```python
from build123d import *

# Parameters (mm, degrees)
F0_R     = 18.25
F0_R_2   = 16.25
F1_DEPTH = 2
F3_DEPTH = 1
F4_R     = 0.99999


# Not quite as in the source:
# - a fillet or chamfer is up to 0.001 mm smaller than in the source, because OpenCascade refuses the exact size


with BuildPart() as f1:
    # F0 (on Top) → F1 (new body)
    with BuildSketch(Plane.XY):
        Circle(F0_R)
        Circle(F0_R_2, mode=Mode.SUBTRACT)
    extrude(amount=F1_DEPTH)

    # F2 (on face) → F3 (join)
    with BuildSketch(Plane.XY.offset(2)):
        with BuildLine():
            ThreePointArc((-13.6956579083, 8.7459393126), (-12.9247475177, 8.70670819), (-12.5275195769, 9.368563064))
            ThreePointArc((-12.5275195769, 9.368563064), (-12.6077000662, 9.7059676033), (-12.8310977719, 9.9712301131))
            ThreePointArc((-12.8310977719, 9.9712301131), (-13.2775195769, 9.368563064), (-13.6956579083, 8.7459393126))
        make_face()
        with BuildLine():
            ThreePointArc((-13.6956579083, 8.7459393126), (-13.2775195769, 9.368563064), (-12.8310977719, 9.9712301131))
            ThreePointArc((-12.8310977719, 9.9712301131), (-13.8903281728, 9.8009582824), (-13.6956579083, 8.7459393126))
        make_face()
        with BuildLine():
            ThreePointArc((-2.0222318148, 16.1236806743), (-2.7640496576, 16.0131986027), (-3.4999795839, 15.8686055755))
            ThreePointArc((-3.4999795839, 15.8686055755), (-2.6914116674, 15.2667244087), (-2.0140496576, 16.0131986027))
            ThreePointArc((-2.0140496576, 16.0131986027), (-2.016097994, 16.0685909213), (-2.0222318148, 16.1236806743))
        make_face()
        with BuildLine():
            ThreePointArc((-2.0222318148, 16.1236806743), (-2.8916211803, 16.7522693075), (-3.4999795839, 15.8686055755))
            ThreePointArc((-3.4999795839, 15.8686055755), (-2.7640496576, 16.0131986027), (-2.0222318148, 16.1236806743))
        make_face()
        with BuildLine():
            ThreePointArc((-15.8686055755, -3.4999795839), (-16.0131986027, -2.7640496576), (-16.1236806743, -2.0222318148))
            ThreePointArc((-16.1236806743, -2.0222318148), (-16.7522693075, -2.8916211803), (-15.8686055755, -3.4999795839))
        make_face()
        with BuildLine():
            ThreePointArc((-15.2631986027, -2.7640496576), (-15.5234851935, -2.1959996802), (-16.1236806743, -2.0222318148))
            ThreePointArc((-16.1236806743, -2.0222318148), (-16.0131986027, -2.7640496576), (-15.8686055755, -3.4999795839))
            ThreePointArc((-15.8686055755, -3.4999795839), (-15.4339988227, -3.2405238067), (-15.2631986027, -2.7640496576))
        make_face()
        with BuildLine():
            ThreePointArc((9.9712301131, 12.8310977719), (9.368563064, 13.2775195769), (8.7459393126, 13.6956579083))
            ThreePointArc((8.7459393126, 13.6956579083), (8.9361678457, 12.664710981), (9.9712301131, 12.8310977719))
        make_face()
        with BuildLine():
            ThreePointArc((10.118563064, 13.2775195769), (9.5871176184, 13.9949691617), (8.7459393126, 13.6956579083))
            ThreePointArc((8.7459393126, 13.6956579083), (9.368563064, 13.2775195769), (9.9712301131, 12.8310977719))
            ThreePointArc((9.9712301131, 12.8310977719), (10.0807780199, 13.0424666965), (10.118563064, 13.2775195769))
        make_face()
        with BuildLine():
            ThreePointArc((-8.618563064, -13.2775195769), (-9.1335101836, -12.565304621), (-9.9712301131, -12.8310977719))
            ThreePointArc((-9.9712301131, -12.8310977719), (-9.368563064, -13.2775195769), (-8.7459393126, -13.6956579083))
            ThreePointArc((-8.7459393126, -13.6956579083), (-8.6511134792, -13.4960741312), (-8.618563064, -13.2775195769))
        make_face()
        with BuildLine():
            ThreePointArc((16.1236806743, 2.0222318148), (16.0131986027, 2.7640496576), (15.8686055755, 3.4999795839))
            ThreePointArc((15.8686055755, 3.4999795839), (15.274127898, 2.6364781349), (16.1236806743, 2.0222318148))
        make_face()
        with BuildLine():
            ThreePointArc((3.4999795839, -15.8686055755), (2.6364781349, -15.274127898), (2.0222318148, -16.1236806743))
            ThreePointArc((2.0222318148, -16.1236806743), (2.7640496576, -16.0131986027), (3.4999795839, -15.8686055755))
        make_face()
        with BuildLine():
            ThreePointArc((13.6956579083, -8.7459393126), (12.664710981, -8.9361678457), (12.8310977719, -9.9712301131))
            ThreePointArc((12.8310977719, -9.9712301131), (13.2775195769, -9.368563064), (13.6956579083, -8.7459393126))
        make_face()
    extrude(amount=-F3_DEPTH)

    # F4 (radius 1 in the source; OpenCascade refuses exactly that, so slightly less here)
    f4_edges = [f1.edges().sort_by_distance(p)[0] for p in [
        (-18.25, 0, 0),
        (-16.25, 0, 0),
    ]]
    fillet(f4_edges, radius=F4_R)


solid = f1.part
```
Model file for the job. Use its own axes, mm. Coordinates: 2 decimals unless noted, no trailing zeros. Order: outer loops, then holes, each group sorted by start corner. A loop starts at its lowest first (then second) coordinate and runs counter-clockwise, first axis right, second up. Notation, with made-up numbers: (65.5, 37) - (116.5, 37) arc R11 ccw to (116.5, 47) - close; hole circle Ø3 at (-14.5, 41.5). An arc over 180 degrees is marked (long way). Return JSON: item names as keys, results as strings. Group by question number.
1) Saw through at C-C, the plane z = 1.5. Write the cut outline in (x, y).
2) Probe line 1 (Y direction, x = 0, z = 1.2); line 2 (X direction, y = -9, z = 1.55); line 3 (Y direction, x = 4.5, z = 1.45). List the from-to ranges inside material, lowest first. Write a range as from..to.
3) Mould opens along Y. For faces 1 (the cylindrical face through (-3.956, -17.816, 1.493)), 2 (the flat face through (-15, -7, 2)), 3 (the flat face through (-15.7, -2.7, 1)) say: released by +Y, released by -Y, zero draft, split by the parting line, or undercut.
4) Flat gauge pins, fed straight in: P1, Ø1.3, axis at x = 13, y = -9.5, coming from the -Z side; P2, Ø1, axis at x = -14, z = 1.5, coming from the +Y side; P3, Ø0.7, axis at x = 3, y = -15.5, coming from the -Z side. Where does each tip first touch, or does it go through?
Values found:
{
 "1": {"outline": "circle Ø36.5 at (0, 0); hole (-16.12, -2.02) arc R0.75 cw to (-15.87, -3.5) arc R16.25 ccw to (-9.97, -12.83) arc R0.75 cw to (-8.75, -13.7) arc R16.25 ccw to (2.02, -16.12) arc R0.75 cw to (3.5, -15.87) arc R16.25 ccw to (12.83, -9.97) arc R0.75 cw to (13.7, -8.75) arc R16.25 ccw to (16.12, 2.02) arc R0.75 cw to (15.87, 3.5) arc R16.25 ccw to (9.97, 12.83) arc R0.75 cw to (8.75, 13.7) arc R16.25 ccw to (-2.02, 16.12) arc R0.75 cw to (-3.5, 15.87) arc R16.25 ccw to (-12.83, 9.97) arc R0.75 cw to (-13.7, 8.75) arc R16.25 ccw to start"},
 "2": {"line 1": "y = -18.25..-16.25, 16.25..18.25", "line 2": "x = -15.88..-13.53, 12.62..15.88", "line 3": "y = -17.69..-15.61, 15.61..17.69"},
 "3": {"face 1": "split by the parting line", "face 2": "zero draft", "face 3": "undercut"},
 "4": {"P1": "stops at z = 0.13", "P2": "stops at y = 12.28", "P3": "stops at z = 1"}
}
